Autodesk Inventor part; units mm, degrees
ref_plane "YZ Plane" through (0, 0, 0) normal (1, 0, 0) x (0, 1, 0)
ref_plane "XZ Plane" through (0, 0, 0) normal (0, 1, 0) x (-1, 0, 0)
ref_plane "XY Plane" through (0, 0, 0) normal (0, 0, 1) x (1, 0, 0)
sketch "Sketch1" plane through (0, 0, 0) normal (0, 0, 1) x (1, 0, 0)
  line L0 (-15, 0) -> (-15, 15) construction
  line L1 (-15, 15) -> (-4.5716, 15) construction
  line L2 (-15, 10.6) -> (-15, 4.4) construction
  line L3 (-15, 10.6) -> (-14.5, 10.6) construction
  line L4 (-14.5, 10.6) -> (-14.5, 11.1)
  line L5 (-14.5, 11.1) -> (-15, 11.1)
  line L6 (-15, 11.1) -> (-15, 10.6) construction
  line L7 (-14.5, 10.6) -> (-13, 10.6)
  line L8 (-15, 15) -> (-15, 11.1)
  line L9 (-13, 13.6) -> (-13, 10.6)
  line L10 (-13, 13.6) -> (-9, 9.6)
  line L11 (-9, 9.6) -> (-9, 7.5)
  line L12 (-15, 7.5) -> (0, 7.5) construction
  line L13 (-9, 7.5) -> (-9, 5.4)
  line L14 (-9, 5.4) -> (-13, 1.4)
  line L15 (-13, 4.4) -> (-13, 1.4)
  line L16 (-15, 4.4) -> (-14.5, 4.4) construction
  line L17 (-14.5, 4.4) -> (-14.5, 3.9)
  line L18 (-14.5, 3.9) -> (-15, 3.9)
  line L19 (-15, 3.9) -> (-15, 4.4) construction
  line L20 (-14.5, 4.4) -> (-13, 4.4)
  line L21 (-4.5716, 15) -> (-5.0716, 15) construction
  line L22 (-5.0716, 15) -> (-5.0716, 14.5)
  line L23 (-5.0716, 14.5) -> (-4.5716, 14.5)
  line L24 (-4.5716, 14.5) -> (-4.5716, 15) construction
  line L25 (-4.5716, 14.5) -> (-4.5716, 13)
  line L26 (-4.5716, 13) -> (-7.5716, 13)
  line L27 (-7.5716, 13) -> (-3.5716, 9)
  line L28 (-3.5716, 9) -> (0, 9)
  line L29 (-15, 3.9) -> (-15, 0)
  line L30 (-15, 0) -> (0, 0)
  line L31 (-4.4, 7) -> (0, 7)
  line L32 (-7, 9.6) -> (-4.4, 7)
  line L33 (-7, 9.6) -> (-7, 4.5716)
  line L34 (-7, 4.5716) -> (-9.5716, 2)
  line L35 (-9.5716, 2) -> (0, 2)
  line L36 (0, 2) -> (0, 0)
  line L37 (0, 9) -> (0, 7)
  line L38 (-15, 15) -> (-5.0716, 15)
  point P0 (-15, 10.85)
  point P1 (-9, 6.45)
  point P2 (-9, 8.55)
  point P3 (-1.7858, 9)
  point P4 (-5.5716, 11)
  dimension "d78" = 15
  dimension "d87" = 6.2
  dimension "d89" = 15
  dimension "d91" = 0.5
  dimension "d92" = 2
  dimension "d93" = 6
  dimension "d96" = 45
  dimension "d97" = 3
  dimension "d98" = 45
  dimension "d121" = 2
  dimension "d122" = 2
  dimension "d124" = 2
  dimension "d126" = 2
  dimension "d127" = 2
extrude "Extrusion1" add sketch "Sketch1" along normal mid plane 100
mirror "Mirror1" about plane through (0, 0, 0) normal (1, 0, 0) of "Extrusion1"
fillet "Fillet1" radius 1 4 edges at (-15, 15, 0) (15, 15, 0) (15, 0, 0) (-15, 0, 0)
fillet "Fillet2" radius 0.5 18 edges at (-13, 13.6, 0) (-9, 9.6, 0) (-9, 5.4, 0) (-13, 1.4, 0) (-7, 9.6, 0) (-7, 4.5716, 0) (-9.5716, 2, 0) (-3.5716, 9, 0) (9, 5.4, 0) (-7.5716, 13, 0) (3.5716, 9, 0) (9.5716, 2, 0) (7, 4.5716, 0) (7.5716, 13, 0) (13, 1.4, 0) (9, 9.6, 0) (13, 13.6, 0) (7, 9.6, 0)
equation "\"d98\" = d96"
properties part number "15mm" material "Aluminum 6061"
Part model, mm, in its own coordinate system. A direction names the side the tool comes from. Round coordinates to 2 decimals unless told otherwise and drop trailing zeros. Write each loop counter-clockwise with the first axis right and the second up, starting at its lowest first coordinate (ties: lowest second). Pieces come first, ordered by that corner, then holes. Notation, with made-up numbers: M 1.5,26.5 L 22.5,26.5 A24 ccw 22.5,54.5 Z; hole C 17,25.25 d5. An arc over 180 degrees is marked long. Return JSON: item names as keys, results as strings. Group by question number.
(1) Pin check, flat tips, straight feed: pin 1 Ø4 at (y, z) = (8, 8) entering from -X; pin 2 Ø4 at (y, z) = (6.5, 15) entering from -X; pin 3 Ø2 at (x, z) = (-0.5, 1) entering from +Y. Stop position of each tip, or through.
(2) Two-plate mould, pull along X, no slides. Class faces 4 (the face through (-5.24, 10.67, -0.7)), 5 (the face through (0, 9, -1)), 6 (the face through (15, 2, -1)), 7 (the face through (-15, 2, -1)): +X half, -X half, draft (parallel to the pull), parting line (faces both ways), or undercut.
(3) Saw through at A-A on x = 1. Write the cut outline in (y, z).
(4) Saw through at B-B on x = -10. Write the cut outline in (y, z).
(5) Which spindle directions (+Z, -Z, +X, -X, +Y, -Y) get a long thin tool onto all of the face, cutting with end or side? Do faces 1 (the face through (9, 7, -1)), 2 (the face through (-15, 13, -1)), 3 (the face through (13, 11, -1)). Say none if no direction does.
(6) Drill centre lines: probe 1 along X at (y, z) = (12.5, 14.5); probe 2 along X at (y, z) = (6, 0); probe 3 along Y at (x, z) = (3, 34). Where is each one in solid material? Low to high.
Returned:
{
 "1": {"pin 1": "x = -9.4", "pin 2": "x = -9.9", "pin 3": "y = 9"},
 "2": {"face 4": "undercut", "face 5": "undercut", "face 6": "+X half", "face 7": "-X half"},
 "3": {"outline": "M 0,-50 L 2,-50 L 2,50 L 0,50 Z; M 7,-50 L 9,-50 L 9,50 L 7,50 Z"},
 "4": {"outline": "M 0,-50 L 4.4,-50 L 4.4,50 L 0,50 Z; M 10.6,-50 L 15,-50 L 15,50 L 10.6,50 Z"},
 "5": {"face 1": "+Z, -Z, +X", "face 2": "+Z, -Z, -X, +Y, -Y", "face 3": "+Z, -Z"},
 "6": {"probe 1": "-15 to -12.99, -11.9 to -6.86, 6.86 to 11.9, 12.99 to 15", "probe 2": "-9 to -7, 7 to 9", "probe 3": "0 to 2, 7 to 9"}
}
